Verification items for the finished model (mm, model axes). Face numbers are marked on the shaded views. A direction names the side the tool comes from. Give positions to 0.01 mm unless a question says otherwise; leave off trailing zeros. Write each loop counter-clockwise with the first axis right and the second up, starting at its lowest first coordinate (ties: lowest second). Pieces come first, ordered by that corner, then holes. Notation, with made-up numbers: M -37,-3 L -22,-3 A16 ccw -22,12 Z; hole C 38.5,63.25 d6. An arc over 180 degrees is marked long. Write item = value, one per line.
from build123d import *

# Parameters (mm, degrees)
SKETCH1_R           = 6.35
SKETCH1_R_2         = 3.96875
BOSS_EXTRUDE1_DEPTH = 7.62
SKETCH2_W           = 4.62
SKETCH2_H           = 1


with BuildPart() as part:
    # Sketch1 → Boss-Extrude1 (new body)
    with BuildSketch(Plane(origin=(0, 0, 0), x_dir=(0, 0, -1), z_dir=(1, 0, 0))):
        with Locations(Location((0, 0, 0), (0, 0, 180))):
            Circle(SKETCH1_R)
        with Locations(Location((0, 0, 0), (0, 0, 180))):
            Circle(SKETCH1_R_2, mode=Mode.SUBTRACT)
    extrude(amount=BOSS_EXTRUDE1_DEPTH)

    # Sketch2 → Cut-Revolve1 (revolve, cut)
    with BuildSketch(Plane.XY, mode=Mode.PRIVATE) as cut_revolve1_sk:
        with Locations((5.31, 5.85)):
            Rectangle(SKETCH2_W, SKETCH2_H)
    revolve(cut_revolve1_sk.sketch.rotate(Axis((7.62, 0, 0), (-1, 0, 0)), 270), axis=Axis((7.62, 0, 0), (-1, 0, 0)), mode=Mode.SUBTRACT)

    # Sketch3 → #60 (0.04) Diameter Hole1 (revolve, cut)
    with BuildSketch(Plane.YZ.offset(1.382942836)):
        Polygon((0, 0), (0, 25.705237194), (0.508, 25.4), (0.508, 0), align=None)
    revolve(axis=Axis((1.382942836, 0, -6.35), (0, 0, 1)), mode=Mode.SUBTRACT)

    # Sketch5 → 1/32 (0.03125) Diameter Hole1 (revolve, cut)
    with BuildSketch(Plane(origin=(1.524, -3.865933193, -5.08), x_dir=(0, 1, 0), z_dir=(1, 0, 0))):
        Polygon((0, 0), (0, 70.342466558), (0.396875, 70.104), (0.396875, 0), align=None)
    revolve(axis=Axis((1.524, -3.865933193, -11.43), (0, 0, 1)), mode=Mode.SUBTRACT)


solid = part.part
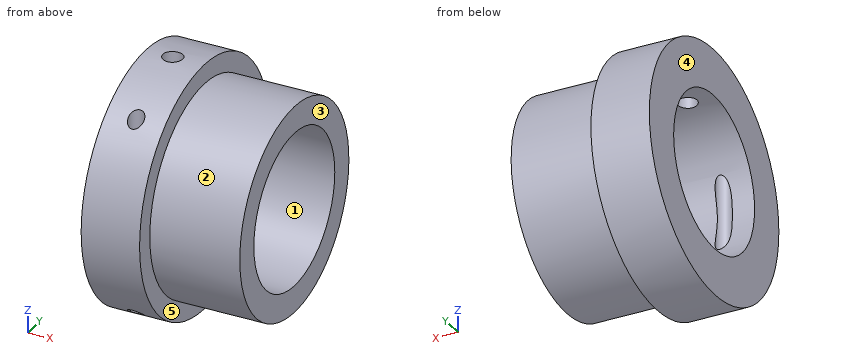
1) Tool access check on the marked faces 4 and 5. Record the directions out of +Z, -Z, +X, -X, +Y, -Y that give a thin tool (end or side, any length) a straight path to the whole face; none if there is none.
From the geometry:
face_4 = +Z, -Z, -X, +Y, -Y
face_5 = +X
2) Cross-section at B-B on z = 4.75. Record the boundary of the cut face in (x, y), plus the area to 3 significant figures.
From the geometry:
outline = M 0,-4.21 L 1.33,-4.21 A0.4 cw long 1.71,-4.21 L 3,-4.21 L 3,-2.46 L 7.62,-2.46 L 7.62,2.46 L 3,2.46 L 3,4.21 L 0,4.21 Z; hole C 1.38,0 d1.02
area = 46.7 mm^2
3) Cross-section at D-D on x = 3.5. Record the boundary of the cut face in (y, z), plus the area to 3 significant figures.
From the geometry:
outline = C 0,0 d10.7; hole C 0,0 d7.94
area = 40.4 mm^2
4) Cross-section at A-A on y = 0. Record the boundary of the cut face in (x, z), plus the area to 3 significant figures.
From the geometry:
outline = M 0,-6.35 L 3,-6.35 L 3,-5.35 L 7.62,-5.35 L 7.62,-3.97 L 0,-3.97 Z; M 0,3.97 L 0.87,3.97 L 0.87,6.35 L 0,6.35 Z; M 1.89,3.97 L 7.62,3.97 L 7.62,5.35 L 3,5.35 L 3,6.35 L 1.89,6.35 Z
area = 24.6 mm^2
5) Depth check by flat-ended pin: P1, Ø4, axis at x = 3.5, y = -0.5, coming from the -Z side; P2, Ø1.5, axis at x = 6, z = -0.5, coming from the +Y side; P3, Ø3, axis at x = 1, z = 4.5, coming from the +Y side; P4, Ø6.5, axis at y = 0, z = 0, coming from the +X side. Enter the tip coordinate at first touch or a pass-through.
From the geometry:
P1 = -6.35
P2 = 5.35
P3 = 5.6
P4 = through
6) Cross-section at C-C on y = 1.75. Record the boundary of the cut face in (x, z), plus the area to 3 significant figures.
From the geometry:
outline = M 0,-6.1 L 3,-6.1 L 3,-5.06 L 7.62,-5.06 L 7.62,-3.56 L 0,-3.56 Z; M 0,3.56 L 7.62,3.56 L 7.62,5.06 L 3,5.06 L 3,6.1 L 0,6.1 Z
area = 29.1 mm^2
7) Material ranges on probe 1 along Y at (x, z) = (4, 0); probe 2 along Z at (x, y) = (4.5, 3); probe 3 along Y at (x, z) = (7.25, -1.5), recorded low to high. Write a range as from..to.
From the geometry:
probe_1 = -5.35..-3.97, 3.97..5.35
probe_2 = -4.43..-2.6, 2.6..4.43
probe_3 = -5.14..-3.67, 3.67..5.14
8) Draft check along Y on the marked faces 1, 2 and 3. Enter one of: +Y half, -Y half, draft (parallel to the pull), parting line (faces both ways), or undercut.
From the geometry:
face_1 = undercut
face_2 = parting line
face_3 = draft
